Source: CAD feature listing. Evaluate the final solid. Frame: model axes, mm. A direction names the side the tool comes from. Coordinates: 2 decimals unless noted, no trailing zeros. Write each loop counter-clockwise with the first axis right and the second up, starting at its lowest first coordinate (ties: lowest second). Pieces come first, ordered by that corner, then holes. Notation, with made-up numbers: (81.25, -14) -> (105.25, -14) arc R9 cw to (105.25, -3) -> close; hole circle Ø10 at (50, -28). An arc over 180 degrees is marked (long way). Write item = value, one per line.
from build123d import *

# Parameters (mm, degrees)
F0_R     = 14.5
F1_DEPTH = 2
F2_R     = 0.4
F3_R     = 1
F4_DEPTH = 1.5
F5_R     = 0.4
F6_R     = 4.5
F7_DEPTH = 1


with BuildPart() as f1:
    # F0 (on Top) → F1 (new body)
    with BuildSketch(Plane.XY):
        Circle(F0_R)
    extrude(amount=F1_DEPTH)

    # F2
    f2_edges = [f1.edges().sort_by_distance(p)[0] for p in [
        (-14.5, 0, 2),
    ]]
    fillet(f2_edges, radius=F2_R)

    # F3 (on face) → F4 (join)
    with BuildSketch(Plane(origin=(0, 0, 0), x_dir=(1, 0, 0), z_dir=(0, 0, -1))):
        with Locations((-10, 0)):
            Circle(F3_R)
        with Locations((10, 0)):
            Circle(F3_R)
    extrude(amount=F4_DEPTH)

    # F5
    f5_edges = [f1.edges().sort_by_distance(p)[0] for p in [
        (-11, 0, -1.5),
        (9, 0, -1.5),
    ]]
    fillet(f5_edges, radius=F5_R)

    # F6 (on face) → F7 (cut)
    with BuildSketch(Plane.XY.offset(2)):
        Circle(F6_R)
    extrude(amount=-F7_DEPTH, mode=Mode.SUBTRACT)


solid = f1.part
1) First-contact query: pin 1 Ø1.5 at (x, z) = (11, 0.5) entering from -Y; pin 2 Ø1.5 at (x, y) = (0, -2.5) entering from -Z; pin 3 Ø1 at (y, z) = (8, 1.5) entering from +X. Flat tips, straight axial feed; report the tip coordinate or a pass-through.
Answer block:
pin_1 = -10.26
pin_2 = 0
pin_3 = 12.41
2) Pull-direction query (Y, two-part tool) for faces 4 (the flat face through (0, 0, 1)), 5 (the cylindrical face through (6.691, -12.864, 0.789)), 6 (the flat face through (-10, 0, -1.5)); classes: +Y half, -Y half, draft (parallel to the pull), parting line (faces both ways), or undercut.
Answer block:
face_4 = undercut
face_5 = parting line
face_6 = draft
3) Cut plane B-B, the plane x = 0. Output: boundary loops of the cut face in (y, z), and give its area (3 significant figures).
Answer block:
outline = (-14.5, 0) -> (14.5, 0) -> (14.5, 1.6) arc R0.4 ccw to (14.1, 2) -> (4.5, 2) -> (4.5, 1) -> (-4.5, 1) -> (-4.5, 2) -> (-14.1, 2) arc R0.4 ccw to (-14.5, 1.6) -> close
area = 48.9 mm2
4) Reachability of faces 1 (the cylindrical face through (-10.8, 0.6, -0.5)), 2 (the cylindrical face through (-0.59, 4.46, 1.51)), 3 (the flat face through (-3.3, 3.3, 2)) from +Z, -Z, +X, -X, +Y, -Y: full face, straight path, thin tool, end or side. Return the list, or none.
Answer block:
face_1 = -Z
face_2 = +Z
face_3 = +Z, +X, -X, +Y, -Y
5) Cut plane A-A, the plane y = 0. Output: boundary loops of the cut face in (x, z), and give its area (3 significant figures).
Answer block:
outline = (-14.5, 0) -> (-11, 0) -> (-11, -1.1) arc R0.4 ccw to (-10.6, -1.5) -> (-9.4, -1.5) arc R0.4 ccw to (-9, -1.1) -> (-9, 0) -> (9, 0) -> (9, -1.1) arc R0.4 ccw to (9.4, -1.5) -> (10.6, -1.5) arc R0.4 ccw to (11, -1.1) -> (11, 0) -> (14.5, 0) -> (14.5, 1.6) arc R0.4 ccw to (14.1, 2) -> (4.5, 2) -> (4.5, 1) -> (-4.5, 1) -> (-4.5, 2) -> (-14.1, 2) arc R0.4 ccw to (-14.5, 1.6) -> close
area = 54.8 mm2
6) Material intervals for probe 1 along Y at (x, z) = (0, 1.65); probe 2 along Z at (x, y) = (0, -2.5); probe 3 along Z at (x, y) = (-8.75, -9.25), sorted ascending. Write a range as [from, to].
Answer block:
probe_1 = [-14.5, -4.5], [4.5, 14.5]
probe_2 = [0, 1]
probe_3 = [0, 2]
